```python
from build123d import *

# Parameters (mm, degrees)
EXTRUDE_1_DEPTH     = 10
SKETCH_2_R          = 1.8
SKETCH_2_R_2        = 1.88
CUT_EXTRUDE_1_DEPTH = 27
SKETCH_3_R          = 4
CUT_EXTRUDE_2_DEPTH = 15
SKETCH_4_W          = 58
SKETCH_4_H          = 2.5
CUT_EXTRUDE_4_DEPTH = 5
SKETCH_5_R          = 2
CUT_EXTRUDE_5_DEPTH = 5


with BuildPart() as part:
    # 草图1 → 凸台-拉伸1 (new body)
    with BuildSketch(Plane.XY):
        with BuildLine():
            Line((-69.33427814, 6.574466706), (-69.33427814, 28.574466706))
            Line((-69.33427814, 28.574466706), (-11.33427814, 28.574466706))
            Line((-11.33427814, 28.574466706), (-11.33427814, 6.574466706))
            Line((-11.33427814, 6.574466706), (-24.33427814, 6.574466706))
            ThreePointArc((-24.33427814, 6.574466706), (-40.33427814, 22.574466706), (-56.33427814, 6.574466706))
            Line((-56.33427814, 6.574466706), (-69.33427814, 6.574466706))
        make_face()
    extrude(amount=EXTRUDE_1_DEPTH)

    # 草图2 → 切除-拉伸1 (cut)
    with BuildSketch(Plane.XZ.offset(-6.574466706)):
        with Locations(Location((-62.83427814, 5, 0), (0, 0, 270))):
            Circle(SKETCH_2_R)
        with Locations(Location((-17.83427814, 5, 0), (0, 0, 270))):
            Circle(SKETCH_2_R_2)
    extrude(amount=-CUT_EXTRUDE_1_DEPTH, mode=Mode.SUBTRACT)

    # 草图3 → 切除-拉伸2 (cut)
    with BuildSketch(Plane(origin=(0, 28.574466706, 0), x_dir=(1, 0, 0), z_dir=(0, 1, 0))):
        with Locations(Location((-62.83427814, -5, 0), (0, 0, 270))):
            Circle(SKETCH_3_R)
        with Locations(Location((-17.83427814, -5, 0), (0, 0, 270))):
            Circle(SKETCH_3_R)
    extrude(amount=-CUT_EXTRUDE_2_DEPTH, mode=Mode.SUBTRACT)

    # 草图4 → 切除-拉伸4 (cut)
    with BuildSketch(Plane(origin=(0, 28.574466706, 0), x_dir=(1, 0, 0), z_dir=(0, 1, 0))):
        with Locations((-40.33427814, -5)):
            Rectangle(SKETCH_4_W, SKETCH_4_H)
    extrude(amount=-CUT_EXTRUDE_4_DEPTH, mode=Mode.SUBTRACT)

    # 草图5 → 切除-拉伸5 (cut)
    with BuildSketch(Plane.XY.offset(10)):
        with Locations((-56.33427814, 25.574466706)):
            Circle(SKETCH_5_R)
        with Locations((-24.33427814, 25.574466706)):
            Circle(SKETCH_5_R)
    extrude(amount=-CUT_EXTRUDE_5_DEPTH, mode=Mode.SUBTRACT)


solid = part.part
```
Model file for the job. Use its own axes, mm. A direction names the side the tool comes from. Coordinates: 2 decimals unless noted, no trailing zeros. Write each loop counter-clockwise with the first axis right and the second up, starting at its lowest first coordinate (ties: lowest second). Pieces come first, ordered by that corner, then holes. Notation, with made-up numbers: (-2, -17) - (37, -17) arc R19 ccw to (37, 12) - close; hole circle Ø11 at (-23, 68). An arc over 180 degrees is marked (long way). Use a Markdown table: item, result. Add a question column.
Item 1: Band-saw the part on B-B, the plane z = 5. Write the cut outline in (x, y).
Item 2: Band-saw the part on D-D, the plane y = 8.5. Write the cut outline in (x, z), and give its area (3 significant figures).
Item 3: Band-saw the part on A-A, the plane y = 15. Write the cut outline in (x, z), and give its area (3 significant figures).
Item 4: Two-plate mould, pull along X, no slides. Class faces 5 (the face through (-11.334, 18, 5)), 6 (the face through (-19, 13.574, 7)), 7 (the face through (-40, 23, 0)): pulls with the +X half, pulls with the -X half, needs draft (parallel to the pull), parting line crosses it, or undercut.
Item 5: Drop flat-ended pins along their axis: pin 1 (2.5 mm diameter, centred on x = -61, z = 4.5, fed in from +Y); pin 2 (1.3 mm diameter, centred on x = -45, z = 5, fed in from +Y); pin 3 (2 mm diameter, centred on x = -62.83, z = 5, fed in from -Y); pin 4 (1.5 mm diameter, centred on x = -31, z = 4.5, fed in from -Y). Give the stop position or say it passes through.
Item 6: 3-axis set-ups, long thin cutter, end or side, ignore diameter. For faces 1 (the face through (-13, 23.574, 5)), 2 (the face through (-16, 6.574, 4)), 3 (the face through (-64, 13.574, 7)), 4 (the face through (-58.332, 25.662, 8.151)): which of +Z, -Z, +X, -X, +Y, -Y reach the whole face in a straight line?
Item 7: Band-saw the part on C-C, the plane z = 8. Write the cut outline in (x, y), and give its area (3 significant figures).
Item 8: Drill centre lines: line 1 along X through (y, z) = (13.75, 3.5); line 2 along X through (y, z) = (14.25, 1.5); line 3 along X through (y, z) = (23, 6). Where is each one in solid material? Low to high.
A:
| question | item | result |
|---|---|---|
| 1 | outline | (-69.33, 6.57) - (-64.63, 6.57) - (-64.63, 13.57) - (-66.83, 13.57) - (-66.83, 23.57) - (-69.33, 23.57) - close; (-61.03, 6.57) - (-56.33, 6.57) arc R16 cw to (-24.33, 6.57) - (-19.71, 6.57) - (-19.71, 13.57) - (-21.83, 13.57) - (-21.83, 23.57) - (-58.83, 23.57) - (-58.83, 13.57) - (-61.03, 13.57) - close; (-15.95, 6.57) - (-11.33, 6.57) - (-11.33, 23.57) - (-13.83, 23.57) - (-13.83, 13.57) - (-15.95, 13.57) - close |
| 2 | outline | (-69.33, 0) - (-56.22, 0) - (-56.22, 10) - (-69.33, 10) - close; (-24.45, 0) - (-11.33, 0) - (-11.33, 10) - (-24.45, 10) - close; hole circle Ø3.6 at (-62.83, 5); hole circle Ø3.76 at (-17.83, 5) |
| 2 | area | 241 mm² |
| 3 | outline | (-69.33, 0) - (-53.94, 0) - (-53.94, 10) - (-69.33, 10) - close; (-26.73, 0) - (-11.33, 0) - (-11.33, 10) - (-26.73, 10) - close; hole circle Ø8 at (-62.83, 5); hole circle Ø8 at (-17.83, 5) |
| 3 | area | 207 mm² |
| 4 | face 5 | pulls with the +X half |
| 4 | face 6 | undercut |
| 4 | face 7 | needs draft |
| 5 | pin 1 | stops at y = 13.57 |
| 5 | pin 2 | stops at y = 23.57 |
| 5 | pin 3 | passes through |
| 5 | pin 4 | stops at y = 19 |
| 6 | face 1 | +X, -X, +Y |
| 6 | face 2 | +Z, -Z, +X, -X, -Y |
| 6 | face 3 | +Y |
| 6 | face 4 | +Z |
| 7 | outline | (-69.33, 6.57) - (-56.33, 6.57) arc R16 cw to (-24.33, 6.57) - (-11.33, 6.57) - (-11.33, 28.57) - (-15.19, 28.57) - (-15.19, 13.57) - (-20.48, 13.57) - (-20.48, 28.57) - (-60.19, 28.57) - (-60.19, 13.57) - (-65.48, 13.57) - (-65.48, 28.57) - (-69.33, 28.57) - close; hole circle Ø4 at (-56.33, 25.57); hole circle Ø4 at (-24.33, 25.57) |
| 7 | area | 690 mm² |
| 8 | line 1 | x = -69.33 to -66.54, -59.13 to -54.64, -26.03 to -21.54, -14.13 to -11.33 |
| 8 | line 2 | x = -69.33 to -64.77, -60.9 to -54.37, -26.3 to -19.77, -15.9 to -11.33 |
| 8 | line 3 | x = -69.33 to -66.71, -58.96 to -21.71, -13.96 to -11.33 |
